```python
from build123d import *

# Parameters (mm, degrees)
SKETCH_1_W           = 50.28
SKETCH_1_H           = 34.2
SKETCH_1_W_2         = 30.28
SKETCH_1_H_2         = 14.2
EXTRUDE_1_DEPTH      = 12.25
SKETCH_4_W           = 13
SKETCH_4_H           = 13.91
EXTRUDE_1_2_DEPTH    = 74.82
SKETCH_5_W           = 13.91
SKETCH_5_H           = 16.23
EXTRUDE_2_DEPTH      = 16
SKETCH_7_R           = 25.25
SKETCH_7_R_2         = 15.25
EXTRUDE_2_2_DEPTH    = 16.23
SKETCH_15_R          = 1.91
CUT_EXTRUDE_6_DEPTH  = 97.964478439
SKETCH_16_W          = 13.91
SKETCH_16_H          = 16.23
EXTRUDE_4_DEPTH      = 10
SKETCH_17_R          = 1.91
CUT_EXTRUDE_7_DEPTH  = 102.16913771
SKETCH_18_W          = 49.344544624
SKETCH_18_H          = 6.125
CUT_EXTRUDE_8_DEPTH  = 105.840616652
SKETCH_19_W          = 34.2
SKETCH_19_H          = 6.125
CUT_EXTRUDE_9_DEPTH  = 10
SKETCH_21_R          = 1.91
CUT_EXTRUDE_10_DEPTH = 10
SKETCH_20_R          = 1.91
CUT_EXTRUDE_11_DEPTH = 10
FILLET_START         = -7.1
FILLET_1_DEPTH       = 14.2
FILLET_2_DEPTH       = 14.2
SKETCH_29_W          = 13.91
SKETCH_29_H          = 74.82
EXTRUDE_5_DEPTH      = 10
SKETCH_30_W          = 10
SKETCH_30_H          = 58.59
CUT_EXTRUDE_13_DEPTH = 102.16913771
SKETCH_32_W          = 34.2
SKETCH_32_H          = 5.745736365
EXTRUDE_6_DEPTH      = 10


with BuildPart() as part:
    # 草圖1 → Extrude 1 (new body)
    with BuildSketch(Plane(origin=(0, 0, 0), x_dir=(1, 0, 0), z_dir=(0, 1, 0))):
        Rectangle(SKETCH_1_W, SKETCH_1_H)
        Rectangle(SKETCH_1_W_2, SKETCH_1_H_2, mode=Mode.SUBTRACT)
    extrude(amount=EXTRUDE_1_DEPTH)

    # 草圖4 → Extrude 1 2 (add)
    with BuildSketch(Plane.XZ):
        with Locations((18.64, 0)):
            Rectangle(SKETCH_4_W, SKETCH_4_H)
    extrude(amount=EXTRUDE_1_2_DEPTH)

    # 草圖5 → Extrude 2 (add)
    with BuildSketch(Plane.ZY.offset(-12.14)):
        with Locations((0, -66.705)):
            Rectangle(SKETCH_5_W, SKETCH_5_H)
    extrude(amount=EXTRUDE_2_DEPTH)

    # 草圖7 → Extrude 2 2 (add)
    with BuildSketch(Plane(origin=(3.626674765, -74.82, 0), x_dir=(1, 0, 0), z_dir=(0, -1, 0))):
        with Locations((-30.978154344, 0)):
            Circle(SKETCH_7_R)
        with Locations((-30.978154344, 0)):
            Circle(SKETCH_7_R_2, mode=Mode.SUBTRACT)
    extrude(amount=-EXTRUDE_2_2_DEPTH)

    # 草圖15 → 除料-伸長6 (cut, through all)
    with BuildSketch(Plane(origin=(0, 0, -6.955), x_dir=(-1, 0, 0), z_dir=(0, 0, -1))):
        with Locations((-4.530883248, -66.705)):
            Circle(SKETCH_15_R)
    extrude(amount=-CUT_EXTRUDE_6_DEPTH, mode=Mode.SUBTRACT)

    # 草圖16 → 填料-伸長4 (add)
    with BuildSketch(Plane(origin=(-60, 0, 0), x_dir=(0, 0, -1), z_dir=(1, 0, 0))):
        with Locations((0, -66.705)):
            Rectangle(SKETCH_16_W, SKETCH_16_H)
    extrude(amount=EXTRUDE_4_DEPTH)

    # 草圖17 → 除料-伸長7 (cut, through all)
    with BuildSketch(Plane(origin=(0, 0, -6.955), x_dir=(-1, 0, 0), z_dir=(0, 0, -1))):
        with Locations((55.812362827, -66.705)):
            Circle(SKETCH_17_R)
    extrude(amount=-CUT_EXTRUDE_7_DEPTH, mode=Mode.SUBTRACT)

    # 草圖18 → 除料-伸長8 (cut, through all)
    with BuildSketch(Plane(origin=(0, 0, -17.1), x_dir=(-1, 0, 0), z_dir=(0, 0, -1))):
        with Locations((0.467727688, 9.1875)):
            Rectangle(SKETCH_18_W, SKETCH_18_H)
    extrude(amount=-CUT_EXTRUDE_8_DEPTH, mode=Mode.SUBTRACT)

    # 草圖19 → 除料-伸長9 (cut)
    with BuildSketch(Plane.ZY.offset(-24.204544624)):
        with Locations((0, 9.1875)):
            Rectangle(SKETCH_19_W, SKETCH_19_H)
    extrude(amount=-CUT_EXTRUDE_9_DEPTH, mode=Mode.SUBTRACT)

    # 草圖21 → 除料-伸長10 (cut)
    with BuildSketch(Plane(origin=(0, 6.125, 0), x_dir=(1, 0, 0), z_dir=(0, 1, 0))):
        with Locations(Location((17.69, 0, 0), (0, 0, 270))):
            Circle(SKETCH_21_R)
    extrude(amount=-CUT_EXTRUDE_10_DEPTH, mode=Mode.SUBTRACT)

    # 草圖20 → 除料-伸長11 (cut)
    with BuildSketch(Plane(origin=(0, 6.125, 0), x_dir=(1, 0, 0), z_dir=(0, 1, 0))):
        with Locations(Location((-17.395, 0, 0), (0, 0, 270))):
            Circle(SKETCH_20_R)
    extrude(amount=-CUT_EXTRUDE_11_DEPTH, mode=Mode.SUBTRACT)

    # 圓角1: read off the stored shape, not the designer's step
    # 圓角1 outline → 圓角1 (cut)
    with BuildSketch(Plane.XY.offset(FILLET_START)):
        with BuildLine():
            add(Edge.make_bspline(
                [(-15.14, 0), (-21.974170252, 5.199829476), (-25.14, 5.745736365)],
                knots=[0, 0, 0, 0.664102345, 0.664102345, 0.664102345], degree=2, weights=[1, 2.223777218, 1.822127795]))
            Line((-15.14, 0), (-15.14, 6.125))
            Line((-15.14, 6.125), (-25.14, 6.125))
            Line((-25.14, 6.125), (-25.14, 5.745736365))
        make_face()
    extrude(amount=FILLET_1_DEPTH, mode=Mode.SUBTRACT)

    # 圓角2: read off the stored shape, not the designer's step
    # 圓角2 outline → 圓角2 (cut)
    with BuildSketch(Plane.XY.offset(FILLET_START)):
        with BuildLine():
            Line((15.14, 6.125), (15.14, 0))
            add(Edge.make_bspline(
                [(15.14, 0), (21.974170252, 5.199829476), (25.14, 5.745736365)],
                knots=[0, 0, 0, 0.664102345, 0.664102345, 0.664102345], degree=2, weights=[1, 2.223777218, 1.822127795]))
            Line((25.14, 5.745736365), (25.14, 6.125))
            Line((25.14, 6.125), (15.14, 6.125))
        make_face()
    extrude(amount=FILLET_2_DEPTH, mode=Mode.SUBTRACT)

    # 草圖29 → 填料-伸長5 (add)
    with BuildSketch(Plane(origin=(25.14, 0, 0), x_dir=(0, 0, -1), z_dir=(1, 0, 0))):
        with Locations((0, -37.41)):
            Rectangle(SKETCH_29_W, SKETCH_29_H)
    extrude(amount=EXTRUDE_5_DEPTH)

    # 草圖30 → 除料-伸長13 (cut, through all)
    with BuildSketch(Plane.XY.offset(6.955)):
        with Locations((17.14, -29.295)):
            Rectangle(SKETCH_30_W, SKETCH_30_H)
    extrude(amount=-CUT_EXTRUDE_13_DEPTH, mode=Mode.SUBTRACT)

    # 草圖32 → 填料-伸長6 (add)
    with BuildSketch(Plane(origin=(25.14, 0, 0), x_dir=(0, 0, -1), z_dir=(1, 0, 0))):
        with Locations((0, 2.872868182)):
            Rectangle(SKETCH_32_W, SKETCH_32_H)
    extrude(amount=EXTRUDE_6_DEPTH)


solid = part.part
```
Here's how the part is built. I have some questions about the finished solid (model axes, mm). A direction names the side the tool comes from. Give positions to 0.01 mm unless a question says otherwise; leave off trailing zeros. Loops run counter-clockwise (first coordinate to the right, second up) from the corner with the lowest first, then second, coordinate; pieces in that order, holes last. Notation, with made-up numbers: M -19,72.5 L 31,72.5 A17 cw 31,94.5 Z; hole C 11.25,-10.5 d11. An arc over 180 degrees is marked long. Return JSON: item names as keys, results as strings.
Item 1: On a 3-axis mill with a long thin cutter (end or side, diameter ignored), from which of +Z, -Z, +X, -X, +Y, -Y can I reach the whole of each face in a straight line? I mean faces 1 (the flat face through (0, 3, -7.1)), 2 (the flat face through (-56, -69, 6.955)), 3 (the flat face through (24, -46, -6.955)), 4 (the flat face through (5, 3, -17.1)). Say none if no direction works.
A:
{"face 1": "+Y", "face 2": "+Z, -X, +Y, -Y", "face 3": "-Z, +X, -Y", "face 4": "-Z, +X, -X, +Y"}
Item 2: Imagine slicing it at A-A on x = 11.5. List the corners of the cut face in (y, z) for me (3 decimals), then the cut area to 3 significant figures.
A:
{"outline": "M -74.82,-6.955 L -58.59,-6.955 L -58.59,6.955 L -74.82,6.955 Z; M 0,-17.1 L 6.125,-17.1 L 6.125,-7.1 L 0,-7.1 Z; M 0,7.1 L 6.125,7.1 L 6.125,17.1 L 0,17.1 Z", "area": "348 mm^2"}
Item 3: Imagine slicing it at D-D on z = 0. State how many separate pieces and enclosed holes the cut face has, then the cut area to 3 significant figures.
A:
{"separate pieces": "5", "enclosed holes": "2", "area": "1,900 mm^2"}
Item 4: I'm going to push flat-ended pins straight in: pin 1 Ø4 at (x, y) = (-55.5, -63) entering from -Z (3 decimals); pin 2 Ø4 at (y, z) = (-19, 1) entering from -X; pin 3 Ø1.8 at (x, y) = (-1.5, 4) entering from +Z. Where does each tip first touch, or does it pass through?
A:
{"pin 1": "stops at z = -6.955", "pin 2": "stops at x = 22.14", "pin 3": "stops at z = 17.1"}
Item 5: Please list where these lines run through material, in increasing order: line 1 (Y direction, x = -10, z = 11.5) (3 decimals); line 2 (Z direction, x = -27, y = -67); line 3 (Z direction, x = 17.69, y = 1.1).
A:
{"line 1": "y = -74.82 to -58.59, 0 to 6.125", "line 2": "z = -25.25 to -15.25, 15.25 to 25.25", "line 3": "z = -17.1 to -1.91, 1.91 to 17.1"}
Item 6: Imagine slicing it at C-C on x = -35. List the corners of the cut face in (y, z) for me, then the cut area to 3 significant figures.
A:
{"outline": "M -74.82,-24.06 L -58.59,-24.06 L -58.59,-13.19 L -74.82,-13.19 Z; M -74.82,13.19 L -58.59,13.19 L -58.59,24.06 L -74.82,24.06 Z", "area": "353 mm^2"}
Item 7: Imagine slicing it at B-B on y = -60. List the corners of the cut face in (x, z) for me (3 decimals).
A:
{"outline": "M -60,-6.955 L -51.625,-6.955 A25.25 ccw -3.078,-6.955 L 35.14,-6.955 L 35.14,6.955 L -3.078,6.955 A25.25 ccw -51.625,6.955 L -60,6.955 Z; hole C -27.351,0 d30.5"}
Item 8: Thinking about a two-plate mould opening in X: for faces 5 (the cylindrical face through (-26.895, -66.819, 25.246)), 6 (the cylindrical face through (-13.264, -66.819, -5.841)), 7 (the flat face through (35.14, -25, 0)), which applies, released by +X, released by -X, zero draft, split by the parting line, or undercut?
A:
{"face 5": "split by the parting line", "face 6": "undercut", "face 7": "released by +X"}
